```python
from build123d import *

# Parameters (mm, degrees)
SKETCH1_W           = 100
SKETCH1_H           = 20.5
SKETCH1_R           = 3.25
SKETCH1_R_2         = 1.5
BOSS_EXTRUDE1_DEPTH = 5
FILLET1_R           = 10.25
CUT_EXTRUDE1_DEPTH  = 10
FILLET2_R           = 10


with BuildPart() as part:
    # Sketch1 → Boss-Extrude1 (new body)
    with BuildSketch(Plane(origin=(0, 0, 0), x_dir=(1, 0, 0), z_dir=(0, 1, 0))):
        with Locations((50, 10.25)):
            Rectangle(SKETCH1_W, SKETCH1_H)
        with Locations(Location((10.25, 10.25, 0), (0, 0, 270))):
            Circle(SKETCH1_R, mode=Mode.SUBTRACT)
        with Locations(Location((17.75, 10.25, 0), (0, 0, 270))):
            Circle(SKETCH1_R_2, mode=Mode.SUBTRACT)
        with Locations(Location((10.25, 17.75, 0), (0, 0, 90))):
            Circle(SKETCH1_R_2, mode=Mode.SUBTRACT)
        with Locations(Location((10.25, 2.75, 0), (0, 0, 90))):
            Circle(SKETCH1_R_2, mode=Mode.SUBTRACT)
        with Locations(Location((2.75, 10.25, 0), (0, 0, 270))):
            Circle(SKETCH1_R_2, mode=Mode.SUBTRACT)
        with Locations(Location((82.25, 10.25, 0), (0, 0, 90))):
            Circle(SKETCH1_R_2, mode=Mode.SUBTRACT)
        with Locations(Location((89.75, 17.75, 0), (0, 0, 270))):
            Circle(SKETCH1_R_2, mode=Mode.SUBTRACT)
        with Locations(Location((89.75, 2.75, 0), (0, 0, 270))):
            Circle(SKETCH1_R_2, mode=Mode.SUBTRACT)
        with Locations(Location((97.25, 10.25, 0), (0, 0, 90))):
            Circle(SKETCH1_R_2, mode=Mode.SUBTRACT)
        with Locations(Location((89.75, 10.25, 0), (0, 0, 90))):
            Circle(SKETCH1_R, mode=Mode.SUBTRACT)
    extrude(amount=BOSS_EXTRUDE1_DEPTH)

    # Fillet1
    fillet1_edges = [part.edges().sort_by_distance(p)[0] for p in [
        (0, 2.5, 0),
        (0, 2.5, -20.5),
        (100, 2.5, -20.5),
        (100, 2.5, 0),
    ]]
    fillet(fillet1_edges, radius=FILLET1_R - 0.0001)  # a hair under: the kernel refuses the full size

    # Sketch2 → Cut-Extrude1 (cut)
    with BuildSketch(Plane(origin=(0, 5, 0), x_dir=(1, 0, 0), z_dir=(0, 1, 0))):
        with BuildLine():
            Line((20.051147892, 13.25), (79.948852108, 13.25))
            ThreePointArc((79.948852108, 13.25), (83.65440733, 18.490524862), (89.75, 20.5))
            Line((89.75, 20.5), (10.25, 20.5))
            ThreePointArc((10.25, 20.5), (16.34559267, 18.490524862), (20.051147892, 13.25))
        make_face()
        with BuildLine():
            Line((20.051147892, 7.25), (79.948852108, 7.25))
            ThreePointArc((79.948852108, 7.25), (83.65440733, 2.009475138), (89.75, 0))
            Line((89.75, 0), (10.25, 0))
            ThreePointArc((10.25, 0), (16.34559267, 2.009475138), (20.051147892, 7.25))
        make_face()
    extrude(amount=-CUT_EXTRUDE1_DEPTH, mode=Mode.SUBTRACT)

    # Fillet2
    fillet2_edges = [part.edges().sort_by_distance(p)[0] for p in [
        (20.051147892, 2.5, -13.25),
        (79.948852108, 2.5, -13.25),
        (79.948852108, 2.5, -7.25),
        (20.051147892, 2.5, -7.25),
    ]]
    fillet(fillet2_edges, radius=FILLET2_R)


solid = part.part
```
Geometry check sheet. Reference: the model listing, model coordinates, mm. A direction names the side the tool comes from. Coordinates: 2 decimals unless noted, no trailing zeros. Order: outer loops, then holes, each group sorted by start corner. A loop starts at its lowest first (then second) coordinate and runs counter-clockwise, first axis right, second up.
Item 1: Section check B-B (z = -6). Enter the section's corners in (x, y), plus the area to 3 significant figures.
Item 2: Mould release check, pull along Z, two halves, no side actions. Record for faces 4 (the cylindrical face through (18.76, 2.46, -11.36)), 5 (the cylindrical face through (14.53, 2.535, -19.564)), 6 (the cylindrical face through (11.714, 2.465, -2.425)), 7 (the cylindrical face through (96.918, 2.535, -2.923)): released by +Z, released by -Z, zero draft, split by the parting line, or undercut.
Item 3: Section check C-C (z = -2.25). Enter the section's corners in (x, y), plus the area to 3 significant figures.
Item 4: Depth check by flat-ended pin: pin 1 (1 mm diameter, centred on y = 3.5, z = -7.5, fed in from +X); pin 2 (3 mm diameter, centred on x = 20.5, y = 4, fed in from +Z); pin 3 (3 mm diameter, centred on x = 72.5, y = 2.5, fed in from -Z). Enter the tip coordinate at first touch or a pass-through.
Item 5: Scan lines: line 1 along Z through (x, y) = (89.75, 2.9); line 2 along X through (y, z) = (0.45, -12); line 3 along Z through (x, y) = (54, 1.65). Record each from-to range of solid material in increasing order.
Item 6: Section check A-A (y = 1.2). Count the separate pieces of the cut face and the enclosed holes in it, plus the area to 3 significant figures.
Item 7: Section check D-D (x = 97.25). Enter the section's corners in (y, z), plus the area to 3 significant figures.
Item 8: Tool access check on faces 1 (the cylindrical face through (78.51, 2.465, -6.285)), 2 (the cylindrical face through (2.923, 2.535, -3.082)), 3 (the cylindrical face through (21.49, 2.465, -14.215)). Record the directions out of +Z, -Z, +X, -X, +Y, -Y that give a thin tool (end or side, any length) a straight path to the whole face; none if there is none.
Check sheet entries:
1. outline: (0.92, 0) - (20.93, 0) - (20.93, 5) - (0.92, 5) - close; (79.07, 0) - (99.08, 0) - (99.08, 5) - (79.07, 5) - close
1. area: 200 mm2
2. face 4: undercut
2. face 5: released by -Z
2. face 6: undercut
2. face 7: released by +Z
3. outline: (3.84, 0) - (8.84, 0) - (8.84, 5) - (3.84, 5) - close; (11.66, 0) - (16.66, 0) - (16.66, 5) - (11.66, 5) - close; (83.34, 0) - (88.34, 0) - (88.34, 5) - (83.34, 5) - close; (91.16, 0) - (96.16, 0) - (96.16, 5) - (91.16, 5) - close
3. area: 99.9 mm2
4. pin 1: stops at x = 99.75
4. pin 2: stops at z = -4.6
4. pin 3: stops at z = -13.25
5. line 1: z = -20.5 to -19.25, -16.25 to -13.5, -7 to -4.25, -1.25 to 0
5. line 2: x = 0.15 to 7.51, 12.99 to 87.01, 92.49 to 99.85
5. line 3: z = -13.25 to -7.25
6. separate pieces: 1
6. enclosed holes: 10
6. area: 910 mm2
7. outline: (0, -17.24) - (5, -17.24) - (5, -11.75) - (0, -11.75) - close; (0, -8.75) - (5, -8.75) - (5, -3.26) - (0, -3.26) - close
7. area: 54.9 mm2
8. face 1: +Z, +Y, -Y
8. face 2: +Z, -X, +Y, -Y
8. face 3: -Z, +Y, -Y
